Design review of the part built by this model. Coordinates are the model's own, in mm. Face numbers are marked on the shaded views. Coordinates: 2 decimals unless noted, no trailing zeros. Write each loop counter-clockwise with the first axis right and the second up, starting at its lowest first coordinate (ties: lowest second). Pieces come first, ordered by that corner, then holes. Notation, with made-up numbers: (-19, -6) - (11, -6) arc R19 ccw to (11, 20) - close; hole circle Ø2 at (5.25, -25). An arc over 180 degrees is marked (long way). Answer as CSV lines item,"result". Start each with the question number.
Q1. We need section B-B (z = 4.5). Write out the cut boundary in (x, y).
Q2. Mouldability with a two-part tool opening along Y and no side actions: class the marked faces 1, 2 and 3 as pulls with the +Y half, pulls with the -Y half, needs draft (parallel to the pull), parting line crosses it, or undercut.
Q3. For line 1 along Y through (x, z) = (0, 15); line 2 along X through (y, z) = (-180, 13); line 3 along Y through (x, z) = (-3.5, 10.5), list the stretches that pass through material, from the lowest coordinate up. Write a range as [from, to].
Q4. Clearance check with flat-ended pins moving along their axes: pin 1 (2 mm diameter, centred on x = 7, y = 160.5, fed in from -Z); pin 2 (6 mm diameter, centred on x = 0.5, z = 15, fed in from -Y); pin 3 (1 mm diameter, centred on x = 2.5, z = 10.5, fed in from +Y); pin 4 (10 mm diameter, centred on x = -7.5, z = 17, fed in from +Y). State where each tip first meets the part, or that it passes through.
Q5. We need section A-A (x = 0). Write out the cut boundary in (y, z).
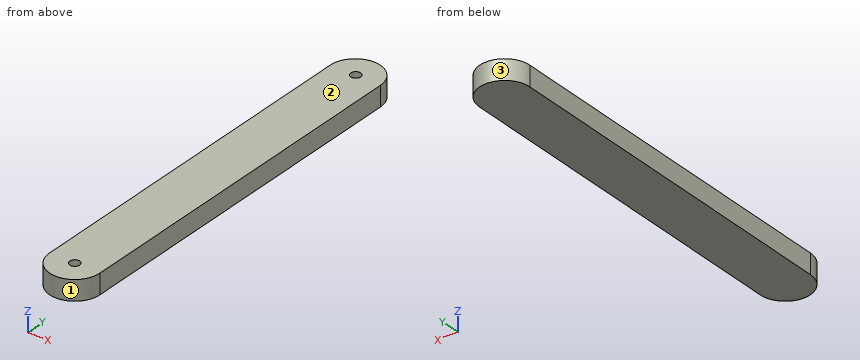
Autodesk Inventor part; units mm, degrees
ref_plane "YZ Plane" through (0, 0, 0) normal (1, 0, 0) x (0, 1, 0)
ref_plane "XZ Plane" through (0, 0, 0) normal (0, 1, 0) x (-1, 0, 0)
ref_plane "XY Plane" through (0, 0, 0) normal (0, 0, 1) x (1, 0, 0)
sketch "Sketch1" plane through (0, 0, 0) normal (0, 0, 1) x (1, 0, 0)
  line L0 (-7.5, 200) -> (7.5, 200)
  line L1 (7.5, 200) -> (7.5, -200)
  line L2 (7.5, -200) -> (-7.5, -200)
  line L3 (-7.5, -200) -> (-7.5, 200)
  line L4 (-35, 0) -> (35, 0)
  line L5 (0, -315) -> (0, 315)
  line L6 (-25, 200) -> (-25, -200)
  line L7 (25, 200) -> (25, -200)
  arc A0 (25, 200) -> (-25, 200) centre (0, 200) ccw
  arc A1 (-25, -200) -> (25, -200) centre (0, -200) ccw
  point P0 (0, 0)
  dimension "d4" = 7.5
  dimension "d5" = 7.5
  dimension "d6" = 200
  dimension "d7" = 200
extrude "Extrusion1" add sketch "Sketch1" along normal blind 20 contours L0 L5 L4 L3 | L0 L1 L4 L5 | L4 L5 L2 L3 | L4 L1 L2 L5
sketch "Sketch2" plane through (0, 0, 20) normal (0, 0, 1) x (1, 0, 0)
  circle A0 centre (0, 180) radius 5
  circle A1 centre (0, -180) radius 5
  line L0 (-10.5, 0) -> (10.5, 0)
  line L1 (0, -280) -> (0, 280)
  point P0 (0, 0)
  dimension "d8" = 10
  dimension "d9" = 180
  dimension "d10" = 180
  dimension "d11" = 10
extrude "Extrusion2" cut sketch "Sketch2" against normal blind 10
sketch "Sketch3" plane through (0, 0, 20) normal (0, 0, 1) x (1, 0, 0)
  circle A0 centre (0, -180) radius 5
  circle A1 centre (0, -180) radius 25
  circle A2 centre (0, 179.3378) radius 25
  line L0 (-25, 179.3378) -> (-25, -180)
  line L1 (25, 179.3378) -> (25, -180)
  point P0 (0, 0)
  dimension "d14" = 50
  dimension "d15" = 50
extrude "Extrusion3" add sketch "Sketch3" against normal blind 20
mirror "Mirror1" about plane through (0, 0, 0) normal (0, 1, 0) of "Extrusion2"
Results list:
1,outline,"(-25, -180) arc R25 ccw to (25, -180) - (25, 179.34) arc R25 ccw to (-25, 179.34) - close"
2,face 1,"pulls with the -Y half"
2,face 2,"needs draft"
2,face 3,"pulls with the +Y half"
3,line 1,"y = [-205, -185], [-175, 175], [185, 204.34]"
3,line 2,"x = [-25, -5], [5, 25]"
3,line 3,"y = [-204.75, -183.57], [-176.43, 176.43], [183.57, 204.09]"
4,pin 1,"stops at z = 0"
4,pin 2,"stops at y = -205"
4,pin 3,"stops at y = 204.26"
4,pin 4,"stops at y = 204.21"
5,outline,"(-205, 0) - (204.34, 0) - (204.34, 20) - (185, 20) - (185, 10) - (175, 10) - (175, 20) - (-175, 20) - (-175, 10) - (-185, 10) - (-185, 20) - (-205, 20) - close"
